Design review of the part built by this model. Coordinates are the model's own, in mm. A direction names the side the tool comes from. Coordinates: 2 decimals unless noted, no trailing zeros. Loops run counter-clockwise (first coordinate to the right, second up) from the corner with the lowest first, then second, coordinate; pieces in that order, holes last. Notation, with made-up numbers: M -21,45.25 L 13,45.25 A25 ccw 13,79.25 Z; hole C 58,-37.5 d1. An arc over 180 degrees is marked long. One line per item, written item: value.
```python
from build123d import *

# Parameters (mm, degrees)
SKETCH1_W           = 70.6882
SKETCH1_H           = 45.974
SKETCH1_R           = 8.0772
BOSS_EXTRUDE1_DEPTH = 6.35
SKETCH2_W           = 70.6882
SKETCH2_H           = 45.974
SKETCH2_W_2         = 45.4406
SKETCH2_H_2         = 20.7264
BOSS_EXTRUDE2_DEPTH = 12.7
SKETCH3_W           = 7.62
SKETCH3_H           = 11.43
CUT_EXTRUDE1_DEPTH  = 12.6238
SKETCH4_W           = 70.6882
SKETCH4_H           = 45.974
SKETCH4_R           = 3.3782
CUT_EXTRUDE2_DEPTH  = 10.16
SKETCH4_3_R         = 3.3782
CUT_EXTRUDE3_DEPTH  = 70.517572708
FILLET1_R           = 5.08


with BuildPart() as part:
    # Sketch1 → Boss-Extrude1 (new body)
    with BuildSketch(Plane(origin=(0, 0, 0), x_dir=(0, 0, -1), z_dir=(1, 0, 0))):
        with Locations((22.6441, 10.287)):
            Rectangle(SKETCH1_W, SKETCH1_H)
        with Locations((35.221300017, 10.287)):
            Circle(SKETCH1_R, mode=Mode.SUBTRACT)
        with Locations((10.066899983, 10.287)):
            Circle(SKETCH1_R, mode=Mode.SUBTRACT)
    extrude(amount=BOSS_EXTRUDE1_DEPTH)

    # Sketch2 → Boss-Extrude2 (add)
    with BuildSketch(Plane.ZY):
        with Locations((-22.6441, 10.287)):
            Rectangle(SKETCH2_W, SKETCH2_H)
        with Locations((-22.6441, 10.287)):
            Rectangle(SKETCH2_W_2, SKETCH2_H_2, mode=Mode.SUBTRACT)
    extrude(amount=BOSS_EXTRUDE2_DEPTH)

    # Sketch3 → Cut-Extrude1 (cut)
    with BuildSketch(Plane(origin=(0, 33.274, 0), x_dir=(1, 0, 0), z_dir=(0, 1, 0))):
        with Locations((-8.89, 22.6441)):
            Rectangle(SKETCH3_W, SKETCH3_H)
    extrude(amount=-CUT_EXTRUDE1_DEPTH, mode=Mode.SUBTRACT)

    # Sketch4 → Cut-Extrude2 (cut)
    # profile 1 of 5: a face of its own
    with BuildSketch(Plane(origin=(6.35, 0, 0), x_dir=(0, 0, -1), z_dir=(1, 0, 0))):
        with Locations((22.6441, 10.287)):
            Rectangle(SKETCH4_W, SKETCH4_H)
        with Locations((-5.715, 26.289)):
            Circle(SKETCH4_R, mode=Mode.SUBTRACT)
        with Locations((-5.715, -5.715)):
            Circle(SKETCH4_R, mode=Mode.SUBTRACT)
        with Locations((51.0032, -5.715)):
            Circle(SKETCH4_R, mode=Mode.SUBTRACT)
        with Locations((51.0032, 26.289)):
            Circle(SKETCH4_R, mode=Mode.SUBTRACT)
        with BuildLine():
            Line((-5.715, 19.685), (-5.715, 0.889))
            ThreePointArc((-5.715, 0.889), (-1.045266817, -1.045266817), (0.889, -5.715))
            Line((0.889, -5.715), (44.3992, -5.715))
            ThreePointArc((44.3992, -5.715), (46.333466817, -1.045266817), (51.0032, 0.889))
            Line((51.0032, 0.889), (51.0032, 19.685))
            ThreePointArc((51.0032, 19.685), (46.333466817, 21.619266817), (44.3992, 26.289))
            Line((44.3992, 26.289), (0.889, 26.289))
            ThreePointArc((0.889, 26.289), (-1.045266817, 21.619266817), (-5.715, 19.685))
        make_face(mode=Mode.SUBTRACT)
    # profile 2 of 5: a face of its own
    with BuildSketch(Plane(origin=(6.35, 0, 0), x_dir=(0, 0, -1), z_dir=(1, 0, 0))):
        with Locations((-5.715, -5.715)):
            Circle(SKETCH4_R)
    # profile 3 of 5: a face of its own
    with BuildSketch(Plane(origin=(6.35, 0, 0), x_dir=(0, 0, -1), z_dir=(1, 0, 0))):
        with Locations((-5.715, 26.289)):
            Circle(SKETCH4_R)
    # profile 4 of 5: a face of its own
    with BuildSketch(Plane(origin=(6.35, 0, 0), x_dir=(0, 0, -1), z_dir=(1, 0, 0))):
        with Locations((51.0032, 26.289)):
            Circle(SKETCH4_R)
    # profile 5 of 5: a face of its own
    with BuildSketch(Plane(origin=(6.35, 0, 0), x_dir=(0, 0, -1), z_dir=(1, 0, 0))):
        with Locations((51.0032, -5.715)):
            Circle(SKETCH4_R)
    extrude(amount=-CUT_EXTRUDE2_DEPTH, mode=Mode.SUBTRACT)

    # Sketch4<3> → Cut-Extrude3 (cut, through all)
    with BuildSketch(Plane(origin=(6.35, 0, 0), x_dir=(0, 0, -1), z_dir=(1, 0, 0))):
        with Locations((-5.715, -5.715)):
            Circle(SKETCH4_3_R)
        with Locations((-5.715, 26.289)):
            Circle(SKETCH4_3_R)
        with Locations((51.0032, 26.289)):
            Circle(SKETCH4_3_R)
        with Locations((51.0032, -5.715)):
            Circle(SKETCH4_3_R)
    extrude(amount=-CUT_EXTRUDE3_DEPTH, mode=Mode.SUBTRACT)

    # Fillet1
    fillet1_edges = [part.edges().sort_by_distance(p)[0] for p in [
        (-8.255, 33.274, 12.7),
        (-8.255, 33.274, -57.9882),
        (-8.255, -12.7, -57.9882),
        (-8.255, -12.7, 12.7),
        (1.27, 19.685, 5.715),
        (1.27, 0.889, 5.715),
        (1.27, -5.715, -0.889),
        (1.27, -5.715, -44.3992),
        (1.27, 0.889, -51.0032),
        (1.27, 19.685, -51.0032),
        (1.27, 26.289, -44.3992),
        (1.27, 26.289, -0.889),
    ]]
    fillet(fillet1_edges, radius=FILLET1_R)


solid = part.part
```
(1) We need section C-C on y = 17.5. State the section outline as (x, z) points.
Reply:
outline: M -12.7,-57.99 L -3.81,-57.99 L -3.81,-50.7 L 6.35,-50.7 L 6.35,-38.86 L 0,-38.86 L 0,-45.36 L -12.7,-45.36 Z; M -12.7,0.08 L 0,0.08 L 0,-6.43 L 6.35,-6.43 L 6.35,5.41 L -3.81,5.41 L -3.81,12.7 L -12.7,12.7 Z; M 0,-31.59 L 6.35,-31.59 L 6.35,-13.7 L 0,-13.7 Z
(2) Insertion check: pin 1 (11 mm diameter, centred on y = -5.72, z = -51, fed in from +X); pin 2 (5.5 mm diameter, centred on y = 24, z = -20, fed in from -X); pin 3 (1 mm diameter, centred on x = 1, y = 2, fed in from +Z). Each pin has a flat end and moves straight along its axis. Give the tip position at first contact, or say it passes through.
Reply:
pin 1: stops at x = -3.81
pin 2: stops at x = -5.08
pin 3: stops at z = 5.16
(3) We need section B-B on x = -8.75. State the section outline as (y, z) points (3 decimals), then the cut area to 3 significant figures.
Reply:
outline: M -12.7,-52.908 A5.08 ccw -7.62,-57.988 L 28.194,-57.988 A5.08 ccw 33.274,-52.908 L 33.274,-28.359 L 20.65,-28.359 L 20.65,-45.364 L -0.076,-45.364 L -0.076,0.076 L 20.65,0.076 L 20.65,-16.929 L 33.274,-16.929 L 33.274,7.62 A5.08 ccw 28.194,12.7 L -7.62,12.7 A5.08 ccw -12.7,7.62 Z; hole C -5.715,-51.003 d6.756; hole C -5.715,5.715 d6.756; hole C 26.289,-51.003 d6.756; hole C 26.289,5.715 d6.756
area: 2,000 mm2
(4) We need section A-A on z = -38.5. State the section outline as (x, y) points (3 decimals).
Reply:
outline: M -12.7,-12.7 L -3.81,-12.7 L -3.81,-5.715 L 6.35,-5.715 L 6.35,2.905 L 0,2.905 L 0,-0.076 L -12.7,-0.076 Z; M -12.7,20.65 L 0,20.65 L 0,17.669 L 6.35,17.669 L 6.35,26.289 L -3.81,26.289 L -3.81,33.274 L -12.7,33.274 Z
(5) To check wall thickness, follow line 1 along Z through (x, y) = (-8, 12); line 2 along Z through (x, y) = (0.75, 17); line 3 along Y through (x, z) = (-11.25, 5). State the ranges of each line that lie inside material, in increasing order. Write a range as [from, to].
Reply:
line 1: z = [-57.99, -45.36], [0.08, 12.7]
line 2: z = [-50.85, -39.71], [-30.73, -14.56], [-5.58, 5.56]
line 3: y = [-12.7, -9.02], [-2.41, 22.99], [29.59, 33.27]
(6) Tool access review of faces 1 (the flat face through (-3.81, -10, -22)), 2 (the flat face through (0, 10, -22)), 3 (the cylindrical face through (1.2, 25.49, -2.07)), 4 (the cylindrical face through (1.34, -1.07, -46.31)), 5 (the flat face through (1, 26.289, -23)): name each direction out of +Z, -Z, +X, -X, +Y, -Y from which nothing blocks a thin tool from reaching the whole face with its end or side.
Reply:
face 1: +X
face 2: -X
face 3: +Z, +X, +Y
face 4: -Z, +X, -Y
face 5: +Z, -Z, +X, +Y
(7) Mouldability with a two-part tool opening along Y and no side actions: class faces 6 (the flat face through (-4.8, 20.65, -23)), 7 (the flat face through (-5.08, 27, -23)), 8 (the cylindrical face through (1.2, 2.14, 4.96)) as released by +Y, released by -Y, zero draft, split by the parting line, or undercut.
Reply:
face 6: undercut
face 7: zero draft
face 8: released by -Y
(8) We need section D-D on x = 1.75. State the section outline as (y, z) points (1 decimal), then the cut area to 3 significant figures.
Reply:
outline: M -5.7,-40.5 A5.1 ccw -2.8,-45.1 A6.6 cw 0.2,-48.1 A5.1 ccw 4.8,-51 L 15.8,-51 A5.1 ccw 20.3,-48.1 A6.6 cw 23.4,-45.1 A5.1 ccw 26.3,-40.5 L 26.3,-4.8 A5.1 ccw 23.4,-0.2 A6.6 cw 20.3,2.8 A5.1 ccw 15.8,5.7 L 4.8,5.7 A5.1 ccw 0.2,2.8 A6.6 cw -2.8,-0.2 A5.1 ccw -5.7,-4.8 Z; hole C 10.3,-35.2 d16.2; hole C 10.3,-10.1 d16.2
area: 1,250 mm2
